Part model, mm, in its own coordinate system. A direction names the side the tool comes from. Give positions to 0.01 mm unless a question says otherwise; leave off trailing zeros. Order: outer loops, then holes, each group sorted by start corner. A loop starts at its lowest first (then second) coordinate and runs counter-clockwise, first axis right, second up. Notation, with made-up numbers: (-24, 86) - (22, 86) arc R18 cw to (22, 103) - close; hole circle Ø7 at (-36.75, 81.25). An arc over 180 degrees is marked (long way). Use one line per item in the form item = value. Start each with the question number.
1. Band-saw the part on D-D, the plane x = 0. State how many separate pieces and enclosed holes the cut face has, plus the area to 3 significant figures.
2. Drill centre lines: line 1 (Z direction, x = -14, y = -10); line 2 (Y direction, x = 38, z = 7.5); line 3 (X direction, y = 13, z = -1). Where is each one in solid material? Low to high.
3. Band-saw the part on B-B, the plane y = 0. List the corners of the cut face in (x, z), plus the area to 3 significant figures.
4. Pull direction X, two halves, no side cores. Call faces 4 (the face through (13.4, 25.4, -2.5)), 5 (the face through (2, 75, -19)): +X half, -X half, draft (parallel to the pull), parting line (faces both ways), or undercut.
5. Band-saw the part on C-C, the plane y = 52.5. List the corners of the cut face in (x, z).
6. Band-saw the part on A-A, the plane x = -38. List the corners of the cut face in (y, z).
7. Tool access for faces 1 (the face through (31.183, -19.168, 10.07)), 2 (the face through (0.28, 53.52, -24.27)), 3 (the face through (0, -20, -1)): list every direction of +Z, -Z, +X, -X, +Y, -Y with a clear straight run to the whole face (end or side of a thin tool).
8. Pin check, flat tips, straight feed: P1, Ø3, axis at y = -9.5, z = 3, coming from the +X side; P2, Ø10, axis at x = -1.5, z = 6, coming from the -Y side; P3, Ø17, axis at x = 3.5, z = 2, coming from the -Y side; P4, Ø1, axis at y = 39.5, z = 6.5, coming from the -X side. Stop position of each tip, or through.
from build123d import *

# Parameters (mm, degrees)
BOSS_EXTRUDE1_DEPTH     = 20
CUT_EXTRUDE1_DEPTH      = 90.721792225
CUT_EXTRUDE1_DEPTH_BACK = 90.721792225
SKETCH2_R               = 15
SKETCH3_R               = 4
BOSS_EXTRUDE2_DEPTH     = 10
SKETCH5_R               = 3.75
BOSS_EXTRUDE3_DEPTH     = 15
CUT_EXTRUDE2_DEPTH      = 110.822584198
CUT_EXTRUDE3_DEPTH      = 105.575331699
SKETCH8_R               = 2.5
CUT_EXTRUDE4_DEPTH      = 115.437756007


with BuildPart() as part:
    # Sketch1 → Boss-Extrude1 (new, symmetric)
    with BuildSketch(Plane(origin=(0, 0, 0), x_dir=(0, 0, -1), z_dir=(1, 0, 0))):
        Polygon((-15, -18.75), (-15, 18.75), (15, 75), (30, 75), (15, 18.75), (15, -18.75), (30, -75), (15, -75), align=None)
    extrude(amount=BOSS_EXTRUDE1_DEPTH, both=True)

    # Sketch2 → Cut-Extrude1 (cut, two sides: drawn at the far end of the back side and taken through both)
    with BuildSketch(Plane.XY.offset(15).offset(-CUT_EXTRUDE1_DEPTH_BACK)):
        Circle(SKETCH2_R)
    extrude(amount=CUT_EXTRUDE1_DEPTH + CUT_EXTRUDE1_DEPTH_BACK, mode=Mode.SUBTRACT)

    # Sketch5 → Boss-Extrude3 (add)
    with BuildSketch(Plane(origin=(0, 75, 0), x_dir=(1, 0, 0), z_dir=(0, 1, 0))):
        with Locations(Location((0, 22.5, 0), (0, 0, 270))):
            Circle(SKETCH5_R)
    boss_extrude3 = extrude(amount=BOSS_EXTRUDE3_DEPTH)

    # Mirror1: Boss-Extrude3 across plane
    add(boss_extrude3.mirror(Plane.ZX))

    # Sketch6 → Cut-Extrude2 (cut, symmetric)
    with BuildSketch(Plane.XY.offset(15)):
        Polygon((20, 18.75), (20, 75), (7.5, 75), align=None)
        Polygon((-20, 75), (-20, 18.75), (-7.5, 75), align=None)
    cut_extrude2 = extrude(amount=CUT_EXTRUDE2_DEPTH, both=True, mode=Mode.SUBTRACT)

    # Mirror2: Cut-Extrude2 across plane
    add(cut_extrude2.mirror(Plane.ZX), mode=Mode.SUBTRACT)

    # Sketch7 → Cut-Extrude3 (cut, symmetric)
    with BuildSketch(Plane.XY):
        with BuildLine():
            Line((-12.107020978, 20), (12.107020978, 20))
            ThreePointArc((12.107020978, 20), (13.667104602, 20.748545213), (14.059395098, 22.433860916))
            Line((14.059395098, 22.433860916), (12.726061765, 28.433860916))
            ThreePointArc((12.726061765, 28.433860916), (12.025142432, 29.560083625), (10.773687644, 30))
            Line((10.773687644, 30), (-10.773687644, 30))
            ThreePointArc((-10.773687644, 30), (-12.025142432, 29.560083625), (-12.726061765, 28.433860916))
            Line((-12.726061765, 28.433860916), (-14.059395098, 22.433860916))
            ThreePointArc((-14.059395098, 22.433860916), (-13.667104602, 20.748545213), (-12.107020978, 20))
        make_face()
        with BuildLine():
            Line((1.884798755, 70), (-1.884798755, 70))
            ThreePointArc((-1.884798755, 70), (-3.136253543, 69.560083625), (-3.837172876, 68.433860916))
            Line((-3.837172876, 68.433860916), (-6.28161732, 57.433860916))
            ThreePointArc((-6.28161732, 57.433860916), (-5.889326824, 55.748545213), (-4.3292432, 55))
            Line((-4.3292432, 55), (4.3292432, 55))
            ThreePointArc((4.3292432, 55), (5.889326824, 55.748545213), (6.28161732, 57.433860916))
            Line((6.28161732, 57.433860916), (3.837172876, 68.433860916))
            ThreePointArc((3.837172876, 68.433860916), (3.136253543, 69.560083625), (1.884798755, 70))
        make_face()
        with BuildLine():
            Line((-8.773687644, 35), (8.773687644, 35))
            ThreePointArc((8.773687644, 35), (10.333771269, 35.748545213), (10.726061765, 37.433860916))
            Line((10.726061765, 37.433860916), (8.28161732, 48.433860916))
            ThreePointArc((8.28161732, 48.433860916), (7.580697987, 49.560083625), (6.3292432, 50))
            Line((6.3292432, 50), (-6.3292432, 50))
            ThreePointArc((-6.3292432, 50), (-7.580697987, 49.560083625), (-8.28161732, 48.433860916))
            Line((-8.28161732, 48.433860916), (-10.726061765, 37.433860916))
            ThreePointArc((-10.726061765, 37.433860916), (-10.333771269, 35.748545213), (-8.773687644, 35))
        make_face()
    cut_extrude3 = extrude(amount=CUT_EXTRUDE3_DEPTH, both=True, mode=Mode.SUBTRACT)

    # Mirror3: Cut-Extrude3 across plane
    add(cut_extrude3.mirror(Plane.ZX), mode=Mode.SUBTRACT)


with BuildPart() as body_2:
    # Sketch3 → Boss-Extrude2 (new body)
    with BuildSketch(Plane.XY.offset(15)):
        with BuildLine():
            ThreePointArc((-20, 20.056349186), (-23.086582838, 15.436951524), (-28.535533906, 16.52081528))
            Line((-28.535533906, 16.52081528), (-33.757359313, 21.742640687))
            ThreePointArc((-33.757359313, 21.742640687), (-40.296100594, 23.043277195), (-44, 17.5))
            Line((-44, 17.5), (-44, -17.5))
            ThreePointArc((-44, -17.5), (-40.296100594, -23.043277195), (-33.757359313, -21.742640687))
            Line((-33.757359313, -21.742640687), (-28.535533906, -16.52081528))
            ThreePointArc((-28.535533906, -16.52081528), (-23.086582838, -15.436951524), (-20, -20.056349186))
            Line((-20, -20.056349186), (-20, -18.75))
            Line((-20, -18.75), (-20, 18.75))
            Line((-20, 18.75), (-20, 20.056349186))
        make_face()
        with Locations((-38, -17.5)):
            Circle(SKETCH3_R, mode=Mode.SUBTRACT)
        with Locations((-38, 17.5)):
            Circle(SKETCH3_R, mode=Mode.SUBTRACT)
    boss_extrude2 = extrude(amount=-BOSS_EXTRUDE2_DEPTH)


with BuildPart() as part_1:
    add(part.part)

    # Mirror6: Boss-Extrude2 across plane
    add(boss_extrude2.mirror(Plane(origin=(0, 0, 0), x_dir=(0, 0, 1), z_dir=(1, 0, 0))))

    # Combine1: union body 2
    add(body_2.part)

    # Sketch8 → Cut-Extrude4 (cut, through all)
    with BuildSketch(Plane(origin=(20, 0, 0), x_dir=(0, 0, -1), z_dir=(1, 0, 0))):
        with Locations((10, 10)):
            Circle(SKETCH8_R)
        with Locations((10, -10)):
            Circle(SKETCH8_R)
    extrude(amount=-CUT_EXTRUDE4_DEPTH, mode=Mode.SUBTRACT)


solid = part_1.part
From the geometry:
q1.separate_pieces = 8
q1.enclosed_holes = 0
q1.area = 1,150 mm²
q2.line_1 = -15 to -12.5, -7.5 to 15
q2.line_2 = -23.5 to -21.5, -13.5 to 13.5, 21.5 to 23.5
q2.line_3 = -20 to -7.48, 7.48 to 20
q3.outline = (-44, 5) - (-20, 5) - (-20, -15) - (-15, -15) - (-15, 15) - (-44, 15) - close; (15, -15) - (20, -15) - (20, 5) - (44, 5) - (44, 15) - (15, 15) - close
q3.area = 780 mm²
q4.face_4 = undercut
q4.face_5 = draft
q5.outline = (-12.5, -24) - (12.5, -24) - (12.5, -3) - (-12.5, -3) - close
q6.outline = (-23.5, 5) - (-21.5, 5) - (-21.5, 15) - (-23.5, 15) - close; (-13.5, 5) - (13.5, 5) - (13.5, 15) - (-13.5, 15) - close; (21.5, 5) - (23.5, 5) - (23.5, 15) - (21.5, 15) - close
q7.face_1 = +Z, -Z, -Y
q7.face_2 = -Z, +X, -X
q7.face_3 = +Z, -Z
q8.P1 = 20
q8.P2 = -35
q8.P3 = -58.31
q8.P4 = through
